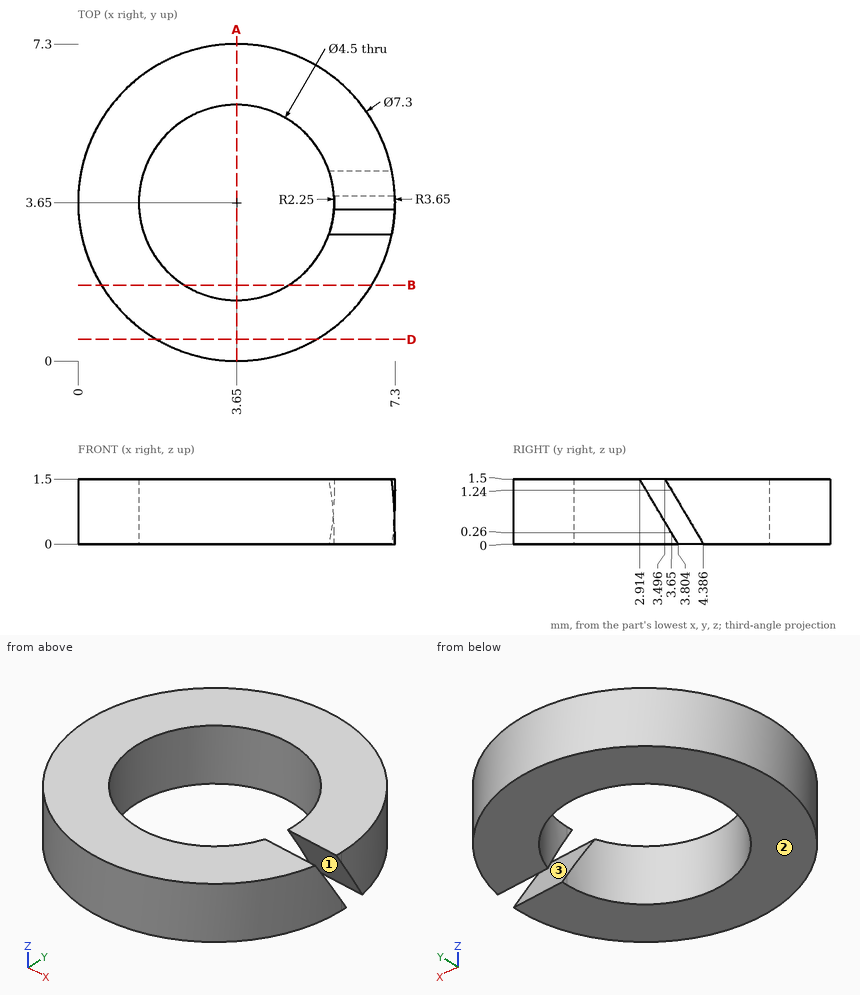
Input: dimensioned drawing with shaded views. Units: mm. Origin: part minimum x, y, z. Round coordinates to 2 decimals unless told otherwise and drop trailing zeros. Loops run counter-clockwise (first coordinate to the right, second up) from the corner with the lowest first, then second, coordinate; pieces in that order, holes last. Notation, with made-up numbers: (49, 71) -> (71, 71) arc R19 ccw to (71, 83) -> close; hole circle Ø4 at (-30, -19). An arc over 180 degrees is marked (long way). Answer as a JSON object with one key per item and string values. Group by question number.
Q1. Section query A-A (x = 3.65). Output: boundary loops of the cut face in (y, z).
Q2. Section query B-B (y = 1.75). Output: boundary loops of the cut face in (x, z) (1 decimal).
Q3. Section query D-D (y = 0.5). Output: boundary loops of the cut face in (x, z).
Q4. Mould query, pull axis Y, two halves, no side actions, for the marked faces 1, 2 and 3. Classes: pulls with the +Y half, pulls with the -Y half, needs draft (parallel to the pull), parting line crosses it, or undercut.
Q5. Contact query for a flat-ended pin moving along its axis: P1, Ø4, axis at x = 4, y = 2.5, coming from the +Z side. Output: stop coordinate, or through.
Q6. Ray query, line 1 (Y direction, x = 3.65, z = 0.55); line 2 (X direction, y = 3.65, z = 0.65). Return the intervals inside material, ascending. Write a range as from..to.
Completed:
{
 "1": {"outline": "(0, 0) -> (1.4, 0) -> (1.4, 1.5) -> (0, 1.5) -> close; (5.9, 0) -> (7.3, 0) -> (7.3, 1.5) -> (5.9, 1.5) -> close"},
 "2": {"outline": "(0.5, 0) -> (2.4, 0) -> (2.4, 1.5) -> (0.5, 1.5) -> close; (4.9, 0) -> (6.8, 0) -> (6.8, 1.5) -> (4.9, 1.5) -> close"},
 "3": {"outline": "(1.81, 0) -> (5.49, 0) -> (5.49, 1.5) -> (1.81, 1.5) -> close"},
 "4": {"face 1": "undercut", "face 2": "needs draft", "face 3": "undercut"},
 "5": {"P1": "z = 1.5"},
 "6": {"line 1": "0..1.4, 5.9..7.3", "line 2": "0..1.4"}
}
